```python
from build123d import *

# Parameters (mm, degrees)
SKETCH1_R               = 12.5
BOSS_EXTRUDE1_DEPTH     = 4
CUT_EXTRUDE1_DEPTH      = 5
CUT_EXTRUDE1_DEPTH_BACK = 5
CHAMFER1_SIZE           = 1
M12_TAPPED_HOLE1_D      = 10.2
M12_TAPPED_HOLE1_DEPTH  = 8


with BuildPart() as part:
    # Sketch1 → Boss-Extrude1 (new body, symmetric)
    with BuildSketch(Plane(origin=(0, 0, 0), x_dir=(1, 0, 0), z_dir=(0, 1, 0))):
        Circle(SKETCH1_R)
    extrude(amount=BOSS_EXTRUDE1_DEPTH, both=True)

    # Sketch2 → Cut-Extrude1 (cut, two sides)
    with BuildSketch(Plane(origin=(0, 0, 0), x_dir=(1, 0, 0), z_dir=(0, 1, 0))) as cut_extrude1_sk:
        with BuildLine():
            ThreePointArc((12.334864981, -2.025118736), (12.499974099, -0.025446565), (12.343007899, 1.974881264))
            Line((12.343007899, 1.974881264), (10.343007899, 1.974881264))
            Line((10.343007899, 1.974881264), (10.343007899, -2.025118736))
            Line((10.343007899, -2.025118736), (12.334864981, -2.025118736))
        make_face()
        with BuildLine():
            ThreePointArc((-2.025118736, -12.334864981), (-0.025446565, -12.499974099), (1.974881264, -12.343007899))
            Line((1.974881264, -12.343007899), (1.974881264, -10.343007899))
            Line((1.974881264, -10.343007899), (-2.025118736, -10.343007899))
            Line((-2.025118736, -10.343007899), (-2.025118736, -12.334864981))
        make_face()
        with BuildLine():
            Line((2.025118736, 10.343007899), (2.025118736, 12.334864981))
            ThreePointArc((2.025118736, 12.334864981), (0.025446565, 12.499974099), (-1.974881264, 12.343007899))
            Line((-1.974881264, 12.343007899), (-1.974881264, 10.343007899))
            Line((-1.974881264, 10.343007899), (2.025118736, 10.343007899))
        make_face()
        with BuildLine():
            ThreePointArc((-12.334864981, 2.025118736), (-12.499974099, 0.025446565), (-12.343007899, -1.974881264))
            Line((-12.343007899, -1.974881264), (-10.343007899, -1.974881264))
            Line((-10.343007899, -1.974881264), (-10.343007899, 2.025118736))
            Line((-10.343007899, 2.025118736), (-12.334864981, 2.025118736))
        make_face()
    extrude(amount=CUT_EXTRUDE1_DEPTH, mode=Mode.SUBTRACT)
    extrude(cut_extrude1_sk.sketch, amount=-CUT_EXTRUDE1_DEPTH_BACK, mode=Mode.SUBTRACT)

    # Chamfer1
    chamfer1_edges = [part.edges().sort_by_distance(p)[0] for p in [
        (8.856809889, 4, -8.820823011),
        (-8.820823011, 4, -8.856809889),
        (-8.856809889, 4, 8.820823011),
        (8.820823011, 4, 8.856809889),
    ]]
    chamfer(chamfer1_edges, length=CHAMFER1_SIZE)

    # M12 Tapped Hole1
    with Locations(Plane(origin=(0, 4, 0), x_dir=(1, 0, 0), z_dir=(0, 1, 0))):
        with Locations((0, 0)):
            Hole(M12_TAPPED_HOLE1_D / 2, depth=M12_TAPPED_HOLE1_DEPTH)


solid = part.part
```
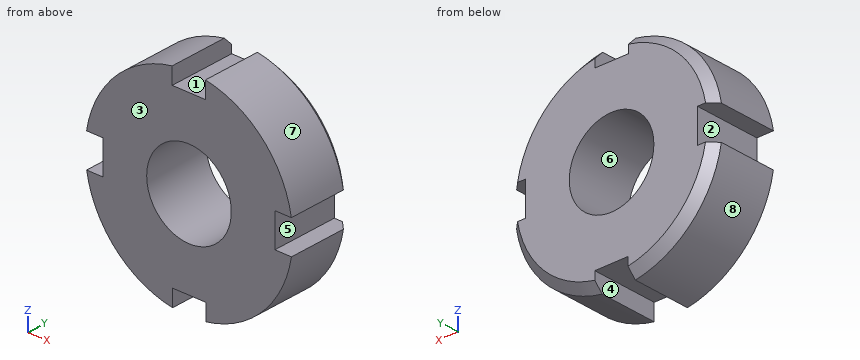
Part model, mm, in its own coordinate system. Face numbers are marked on the shaded views. A direction names the side the tool comes from. Round coordinates to 2 decimals unless told otherwise and drop trailing zeros. Write each loop counter-clockwise with the first axis right and the second up, starting at its lowest first coordinate (ties: lowest second). Pieces come first, ordered by that corner, then holes.
Item 1: Which spindle directions (+Z, -Z, +X, -X, +Y, -Y) get a long thin tool onto all of the face, cutting with end or side? Do the marked faces 1, 2, 3, 4 and 5. Say none if no direction does.
Results:
face 1: +Z, +Y, -Y
face 2: -X, +Y, -Y
face 3: +Z, -Z, +X, -X, -Y
face 4: -Z, +Y, -Y
face 5: +X, +Y, -Y
Item 2: Cut at A-A, the plane z = 0. Give the cut face in (x, y).
Results:
outline: (-10.34, -4) - (-5.1, -4) - (-5.1, 4) - (-10.34, 4) - close; (5.1, -4) - (10.34, -4) - (10.34, 4) - (5.1, 4) - close
Item 3: Drop flat-ended pins along their axis: pin 1 Ø2 at (y, z) = (-1, 11) entering from -X; pin 2 Ø2 at (y, z) = (2, 11) entering from +X; pin 3 Ø2 at (y, z) = (1, -4) entering from -X. Give the stop position or say it passes through.
Results:
pin 1: stops at x = -7.5
pin 2: stops at x = 7.5
pin 3: stops at x = -12.13
Item 4: Two-plate mould, pull along X, no slides. Class the marked faces 6, 7 and 8: +X half, -X half, draft (parallel to the pull), parting line (faces both ways), or undercut.
Results:
face 6: undercut
face 7: +X half
face 8: -X half
Item 5: Cut at B-B, the plane y = 2.5. Give the cut face in (x, z).
Results:
outline: (-12.34, 1.97) - (-10.34, 1.97) - (-10.34, -2.03) - (-12.33, -2.03) arc R12.5 ccw to (-1.97, -12.34) - (-1.97, -10.34) - (2.03, -10.34) - (2.03, -12.33) arc R12.5 ccw to (12.34, -1.97) - (10.34, -1.97) - (10.34, 2.03) - (12.33, 2.03) arc R12.5 ccw to (1.97, 12.34) - (1.97, 10.34) - (-2.03, 10.34) - (-2.03, 12.33) arc R12.5 ccw to start; hole circle Ø10.2 at (0, 0)
Item 6: Probe L1, parallel to Z at x = 0, y = 0.5; L2, parallel to X at y = 2.75, z = 0.25; L3, parallel to Z at x = 10.5, y = 1. List the from-to ranges inside material, lowest first.
Results:
L1: z = -10.34 to -5.1, 5.1 to 10.34
L2: x = -10.34 to -5.09, 5.09 to 10.34
L3: z = -6.78 to -1.97, 2.03 to 6.78
Item 7: Cut at C-C, the plane x = 0. Give the cut face in (y, z).
Results:
outline: (-4, -10.34) - (4, -10.34) - (4, -5.1) - (-4, -5.1) - close; (-4, 5.1) - (4, 5.1) - (4, 10.34) - (-4, 10.34) - close
